from build123d import *

# Parameters (mm, degrees)
F0_R      = 9
F1_DEPTH  = 40
F3_R      = 9
F4_R      = 8
F6_R      = 8
F8_DEPTH  = 39
F9_R      = 9
F9_R_2    = 8
F10_DEPTH = 45
F12_DEPTH = 20
F13_W     = 4
F13_H     = 4
F14_DEPTH = 100
F7_R      = 7
F15_DEPTH = 25
F16_SIZE2 = 0.99999
F16_SIZE  = 0.99999


# Not quite as in the source:
# - a fillet or chamfer is up to 0.001 mm smaller than in the source, because OpenCascade refuses the exact size


with BuildPart() as f1:
    # F0 (on Top) → F1 (new body)
    with BuildSketch(Plane.XY):
        Circle(F0_R)
    extrude(amount=F1_DEPTH)

    # F3 (on face) → F5 section 0
    with BuildSketch(Plane.XY.offset(40)):
        Circle(F3_R)
    # F4 (on offset) → F5 section 1
    with BuildSketch(Plane.XY.offset(42)):
        Circle(F4_R)
    loft()

    # F6 (on face) → F8 (cut)
    with BuildSketch(Plane(origin=(0, 0, 0), x_dir=(1, 0, 0), z_dir=(0, 0, -1))):
        Circle(F6_R)
    extrude(amount=-F8_DEPTH, mode=Mode.SUBTRACT)

    # F9 (on face) → F10 (join)
    with BuildSketch(Plane(origin=(0, 0, 0), x_dir=(1, 0, 0), z_dir=(0, 0, -1))):
        Circle(F9_R)
        Circle(F9_R_2, mode=Mode.SUBTRACT)
    extrude(amount=F10_DEPTH)

    # F11 (on face) → F12 (cut)
    with BuildSketch(Plane(origin=(0, 0, -45), x_dir=(1, 0, 0), z_dir=(0, 0, -1))):
        with BuildLine():
            ThreePointArc((0, -9), (6.3639610307, -6.3639610307), (9, 0))
            ThreePointArc((9, 0), (6.3639610307, 6.3639610307), (0, 9))
            Line((0, 9), (0, 8))
            ThreePointArc((0, 8), (5.6568542495, 5.6568542495), (8, 0))
            ThreePointArc((8, 0), (5.6568542495, -5.6568542495), (0, -8))
            Line((0, -8), (0, -9))
        make_face()
    extrude(amount=-F12_DEPTH, mode=Mode.SUBTRACT)

    # F13 (on face) → F14 (cut)
    with BuildSketch(Plane(origin=(0, 0, -25), x_dir=(1, 0, 0), z_dir=(0, 0, -1))):
        with Locations((8, 0)):
            Rectangle(F13_W, F13_H)
    extrude(amount=-F14_DEPTH, mode=Mode.SUBTRACT)

    # F7 (on face) → F15 (cut)
    with BuildSketch(Plane.XY.offset(42)):
        Circle(F7_R)
    extrude(amount=-F15_DEPTH, mode=Mode.SUBTRACT)

    # F16 (size 1 and 1 in the source; OpenCascade refuses exactly that, so slightly less here)
    f16_edges = [f1.edges().sort_by_distance(p)[0] for p in [
        (-7, 0, 39),
    ]]
    chamfer(f16_edges, length=F16_SIZE, length2=F16_SIZE2)


solid = f1.part
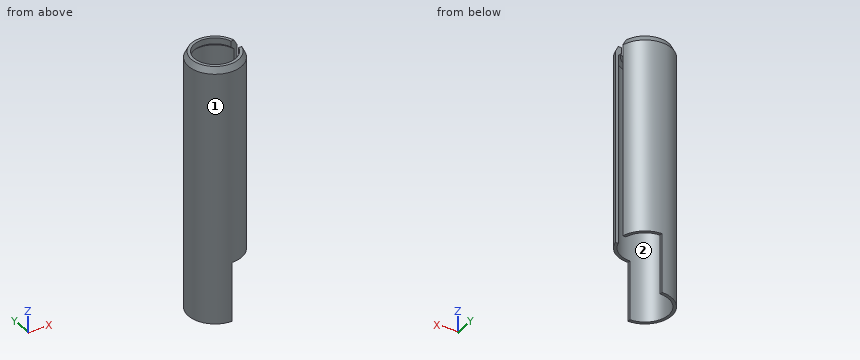
The listing builds one solid part. Answer for the finished solid, in the listing's coordinates (mm). Face numbers are marked on the shaded views. Give positions to 0.01 mm unless a question says otherwise; leave off trailing zeros. Order: outer loops, then holes, each group sorted by start corner. A loop starts at its lowest first (then second) coordinate and runs counter-clockwise, first axis right, second up. Notation, with made-up numbers: (-23.75, 85) -> (26.25, 85) arc R20 cw to (26.25, 111) -> close; hole circle Ø6 at (77, 6). An arc over 180 degrees is marked (long way). Put each result on its own line as item: value.
Item 1: For a pull along X with two mould halves and no side action, classify the marked faces 1 and 2 as released by +X, released by -X, zero draft, split by the parting line, or undercut.
Established:
face 1: split by the parting line
face 2: undercut
Item 2: A cutting plane is placed at B-B on z = -16. Give the vertices of the cut face in (x, y).
Established:
outline: (7.75, -2) arc R8 cw (long way) to (7.75, 2) -> (8.77, 2) arc R9 ccw (long way) to (8.77, -2) -> close
Item 3: Given P1, Ø5.5, axis at x = 5.5, y = 7, coming from the -Z side; P2, Ø1.5, axis at x = 7, z = -23, coming from the +Y side; P3, Ø3, axis at y = -4.5, z = 22, coming from the -X side; P4, Ø5, axis at x = -3, y = 1.5, coming from the +Z side, each flat-ended and moving along its own axis, determine where each tip first touches the part or whether it passes through.
Established:
P1: stops at z = -25
P2: stops at y = 6.48
P3: stops at x = -8.49
P4: passes through
Item 4: A cutting plane is placed at A-A on z = -29. Give the vertices of the cut face in (x, y), plus the area to 3 significant figures.
Established:
outline: (0, -9) -> (0, -8) arc R8 cw to (0, 8) -> (0, 9) arc R9 ccw to start
area: 26.7 mm^2
Item 5: Straight lines are drawn through the part: line 1 (Y direction, x = 0, z = 10); line 2 (X direction, y = 0, z = -7.5); line 3 (Y direction, x = -6.5, z = -39). For each, find the intervals that lie inside material, in ascending order.
Established:
line 1: y = -9 to -8, 8 to 9
line 2: x = -9 to -8
line 3: y = -6.22 to -4.66, 4.66 to 6.22
